CAD build for the part. Positions are in the model's coordinates, mm. Face numbers are marked on the shaded views. A direction names the side the tool comes from. Coordinates: 2 decimals unless noted, no trailing zeros. Write each loop counter-clockwise with the first axis right and the second up, starting at its lowest first coordinate (ties: lowest second). Pieces come first, ordered by that corner, then holes. Notation, with made-up numbers: (-2, -16) - (36, -16) arc R11 ccw to (36, 2) - close; hole circle Ø1 at (49, -10). An arc over 180 degrees is marked (long way). Answer in a Markdown table with one row per item. Add a question column.
Q1. Band-saw the part on D-D (x = -22). List the corners of the cut face in (y, z), and give its area (3 significant figures).
Q2. Pin check, flat tips, straight feed: pin 1 (1 mm diameter, centred on x = 2.5, y = -6.5, fed in from -Z); pin 2 (1 mm diameter, centred on y = -7, z = -6, fed in from -X); pin 3 (4 mm diameter, centred on y = -4.5, z = -5.5, fed in from +X); pin 4 (2.5 mm diameter, centred on x = 0, z = 24.28, fed in from -Y). Stop position of each tip, or through.
Q3. Band-saw the part on A-A (x = 0). List the corners of the cut face in (y, z).
Q4. Band-saw the part on C-C (y = -5.25). State how many separate pieces and enclosed holes the cut face has, and give its area (3 significant figures).
Q5. Two-plate mould, pull along Z, no slides. Class the marked faces 1, 2 and 3: +Z half, -Z half, draft (parallel to the pull), parting line (faces both ways), or undercut.
Q6. Drill centre lines: line 1 along Z through (x, y) = (0, -3); line 2 along Z through (x, y) = (-39, -7.25). Where is each one in solid material? Low to high. Write a range as from..to.
Q7. 3-axis set-ups, long thin cutter, end or side, ignore diameter. For the marked faces 4, 5, 6 and 7: which of +Z, -Z, +X, -X, +Y, -Y reach the whole face in a straight line?
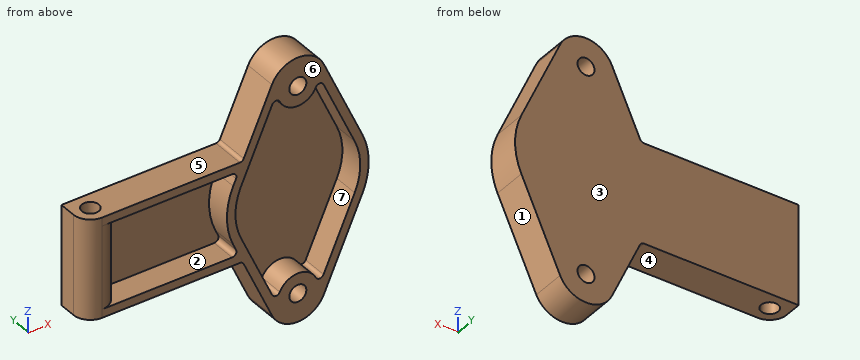
```python
from build123d import *

# Parameters (mm, degrees)
F0_R     = 2
F1_DEPTH = 8
F2_DEPTH = 2
F3_R     = 1
F5_D     = 4
F6_R     = 3.99999


# Not quite as in the source:
# - a fillet or chamfer is up to 0.001 mm smaller than in the source, because OpenCascade refuses the exact size
# - a feature names something its author has since deleted; it is built from what else it names


with BuildPart() as f1:
    # F0 (on Front) → F1 (new body)
    with BuildSketch(Plane.XZ):
        with BuildLine():
            Line((15.1970139668, 6.8636525628), (6.0880650012, 27.0320429916))
            ThreePointArc((6.0880650012, 27.0320429916), (0, 30.9626), (-6.0880650012, 27.0320429916))
            Line((-6.0880650012, 27.0320429916), (-12.9901204821, 11.75))
            Line((-12.9901204821, 11.75), (-13.8934101123, 9.75))
            Line((-13.8934101123, 9.75), (-15.1970139668, 6.8636525628))
            ThreePointArc((-15.1970139668, 6.8636525628), (-16.6751, 0), (-15.1970139668, -6.8636525628))
            Line((-15.1970139668, -6.8636525628), (-13.8934101123, -9.75))
            Line((-13.8934101123, -9.75), (-12.9901204821, -11.75))
            Line((-12.9901204821, -11.75), (-6.0880650012, -27.0320429916))
            ThreePointArc((-6.0880650012, -27.0320429916), (0, -30.9626), (6.0880650012, -27.0320429916))
            Line((6.0880650012, -27.0320429916), (15.1970139668, -6.8636525628))
            ThreePointArc((15.1970139668, -6.8636525628), (16.6751, 0), (15.1970139668, 6.8636525628))
        make_face()
        with Locations((0, -24.2824)):
            Circle(F0_R, mode=Mode.SUBTRACT)
        with BuildLine():
            Line((-13.3742945868, 6.0404308054), (-6.0462846285, 22.2655920687))
            ThreePointArc((-6.0462846285, 22.2655920687), (-5.1436901116, 22.8539427752), (-4.2309206889, 22.2815046593))
            ThreePointArc((-4.2309206889, 22.2815046593), (0, 19.6022), (4.2309206889, 22.2815046593))
            ThreePointArc((4.2309206889, 22.2815046593), (5.1436901116, 22.8539427752), (6.0462846285, 22.2655920687))
            Line((6.0462846285, 22.2655920687), (13.3742945868, 6.0404308054))
            ThreePointArc((13.3742945868, 6.0404308054), (14.6751, 0), (13.3742945868, -6.0404308054))
            Line((13.3742945868, -6.0404308054), (6.0462846285, -22.2655920687))
            ThreePointArc((6.0462846285, -22.2655920687), (5.1436901116, -22.8539427752), (4.2309206889, -22.2815046593))
            ThreePointArc((4.2309206889, -22.2815046593), (0, -19.6022), (-4.2309206889, -22.2815046593))
            ThreePointArc((-4.2309206889, -22.2815046593), (-5.1436901116, -22.8539427752), (-6.0462846285, -22.2655920687))
            Line((-6.0462846285, -22.2655920687), (-13.3742945868, -6.0404308054))
            ThreePointArc((-13.3742945868, -6.0404308054), (-14.6751, 0), (-13.3742945868, 6.0404308054))
        make_face(mode=Mode.SUBTRACT)
        with Locations((0, 24.2824)):
            Circle(F0_R, mode=Mode.SUBTRACT)
        Polygon((-13.8934101123, 9.75), (-12.9901204821, 11.75), (-50, 11.75), (-50, -11.75), (-12.9901204821, -11.75), (-13.8934101123, -9.75), (-42, -9.75), (-42, 9.75), align=None)
    extrude(amount=F1_DEPTH)

    # F0 (on Front) → F2 (join)
    with BuildSketch(Plane.XZ):
        with BuildLine():
            Line((15.1970139668, 6.8636525628), (6.0880650012, 27.0320429916))
            ThreePointArc((6.0880650012, 27.0320429916), (0, 30.9626), (-6.0880650012, 27.0320429916))
            Line((-6.0880650012, 27.0320429916), (-12.9901204821, 11.75))
            Line((-12.9901204821, 11.75), (-13.8934101123, 9.75))
            Line((-13.8934101123, 9.75), (-15.1970139668, 6.8636525628))
            ThreePointArc((-15.1970139668, 6.8636525628), (-16.6751, 0), (-15.1970139668, -6.8636525628))
            Line((-15.1970139668, -6.8636525628), (-13.8934101123, -9.75))
            Line((-13.8934101123, -9.75), (-12.9901204821, -11.75))
            Line((-12.9901204821, -11.75), (-6.0880650012, -27.0320429916))
            ThreePointArc((-6.0880650012, -27.0320429916), (0, -30.9626), (6.0880650012, -27.0320429916))
            Line((6.0880650012, -27.0320429916), (15.1970139668, -6.8636525628))
            ThreePointArc((15.1970139668, -6.8636525628), (16.6751, 0), (15.1970139668, 6.8636525628))
        make_face()
        with Locations((0, -24.2824)):
            Circle(F0_R, mode=Mode.SUBTRACT)
        with BuildLine():
            Line((-13.3742945868, 6.0404308054), (-6.0462846285, 22.2655920687))
            ThreePointArc((-6.0462846285, 22.2655920687), (-5.1436901116, 22.8539427752), (-4.2309206889, 22.2815046593))
            ThreePointArc((-4.2309206889, 22.2815046593), (0, 19.6022), (4.2309206889, 22.2815046593))
            ThreePointArc((4.2309206889, 22.2815046593), (5.1436901116, 22.8539427752), (6.0462846285, 22.2655920687))
            Line((6.0462846285, 22.2655920687), (13.3742945868, 6.0404308054))
            ThreePointArc((13.3742945868, 6.0404308054), (14.6751, 0), (13.3742945868, -6.0404308054))
            Line((13.3742945868, -6.0404308054), (6.0462846285, -22.2655920687))
            ThreePointArc((6.0462846285, -22.2655920687), (5.1436901116, -22.8539427752), (4.2309206889, -22.2815046593))
            ThreePointArc((4.2309206889, -22.2815046593), (0, -19.6022), (-4.2309206889, -22.2815046593))
            ThreePointArc((-4.2309206889, -22.2815046593), (-5.1436901116, -22.8539427752), (-6.0462846285, -22.2655920687))
            Line((-6.0462846285, -22.2655920687), (-13.3742945868, -6.0404308054))
            ThreePointArc((-13.3742945868, -6.0404308054), (-14.6751, 0), (-13.3742945868, 6.0404308054))
        make_face(mode=Mode.SUBTRACT)
        with Locations((0, 24.2824)):
            Circle(F0_R, mode=Mode.SUBTRACT)
        with BuildLine():
            ThreePointArc((-4.2309206889, 22.2815046593), (-5.1436901116, 22.8539427752), (-6.0462846285, 22.2655920687))
            Line((-6.0462846285, 22.2655920687), (-13.3742945868, 6.0404308054))
            ThreePointArc((-13.3742945868, 6.0404308054), (-14.6751, 0), (-13.3742945868, -6.0404308054))
            Line((-13.3742945868, -6.0404308054), (-6.0462846285, -22.2655920687))
            ThreePointArc((-6.0462846285, -22.2655920687), (-5.1436901116, -22.8539427752), (-4.2309206889, -22.2815046593))
            ThreePointArc((-4.2309206889, -22.2815046593), (0, -19.6022), (4.2309206889, -22.2815046593))
            ThreePointArc((4.2309206889, -22.2815046593), (5.1436901116, -22.8539427752), (6.0462846285, -22.2655920687))
            Line((6.0462846285, -22.2655920687), (13.3742945868, -6.0404308054))
            ThreePointArc((13.3742945868, -6.0404308054), (14.6751, 0), (13.3742945868, 6.0404308054))
            Line((13.3742945868, 6.0404308054), (6.0462846285, 22.2655920687))
            ThreePointArc((6.0462846285, 22.2655920687), (5.1436901116, 22.8539427752), (4.2309206889, 22.2815046593))
            ThreePointArc((4.2309206889, 22.2815046593), (0, 19.6022), (-4.2309206889, 22.2815046593))
        make_face()
        with BuildLine():
            Line((-15.1970139668, 6.8636525628), (-13.8934101123, 9.75))
            Line((-13.8934101123, 9.75), (-42, 9.75))
            Line((-42, 9.75), (-42, -9.75))
            Line((-42, -9.75), (-13.8934101123, -9.75))
            Line((-13.8934101123, -9.75), (-15.1970139668, -6.8636525628))
            ThreePointArc((-15.1970139668, -6.8636525628), (-16.6751, 0), (-15.1970139668, 6.8636525628))
        make_face()
    extrude(amount=F2_DEPTH)

    # F3
    f3_edges = [f1.edges().sort_by_distance(p)[0] for p in [
        (-13.89341, -5, -9.75),
        (-12.99012, -4, -11.75),
        (-13.89341, -5, 9.75),
        (-12.99012, -4, 11.75),
    ]]
    fillet(f3_edges, radius=F3_R)

    # F5 (through all)
    with Locations(Plane.XY.offset(11.75)):
        with Locations((-46, -4)):
            Hole(F5_D / 2)

    # F6 (radius 4 in the source; OpenCascade refuses exactly that, so slightly less here)
    f6_edges = [f1.edges().sort_by_distance(p)[0] for p in [
        (-50, -8, 0),
        (-42, -8, 0),
    ]]
    fillet(f6_edges, radius=F6_R)


solid = f1.part
```
Checked values:
| question | item | result |
|---|---|---|
| 1 | outline | (-8, -11.75) - (0, -11.75) - (0, 11.75) - (-8, 11.75) - (-8, 9.75) - (-2, 9.75) - (-2, -9.75) - (-8, -9.75) - close |
| 1 | area | 71.0 mm² |
| 2 | pin 1 | stops at z = -30.66 |
| 2 | pin 2 | stops at x = -49.12 |
| 2 | pin 3 | stops at x = 16.3 |
| 2 | pin 4 | passes through |
| 3 | outline | (-8, -30.96) - (0, -30.96) - (0, -26.28) - (-8, -26.28) - close; (-8, -22.28) - (0, -22.28) - (0, 22.28) - (-8, 22.28) - (-8, 19.6) - (-2, 19.6) - (-2, -19.6) - (-8, -19.6) - close; (-8, 26.28) - (0, 26.28) - (0, 30.96) - (-8, 30.96) - close |
| 4 | separate pieces | 2 |
| 4 | enclosed holes | 4 |
| 4 | area | 623 mm² |
| 5 | face 1 | -Z half |
| 5 | face 2 | undercut |
| 5 | face 3 | draft |
| 6 | line 1 | z = -30.96..-26.28, -22.28..-19.6, 19.6..22.28, 26.28..30.96 |
| 6 | line 2 | z = -11.75..-9.75, 9.75..11.75 |
| 7 | face 4 | -Z, -X, +Y, -Y |
| 7 | face 5 | +Z, -X, +Y, -Y |
| 7 | face 6 | +Z, -Z, +X, -X, -Y |
| 7 | face 7 | -Y |
